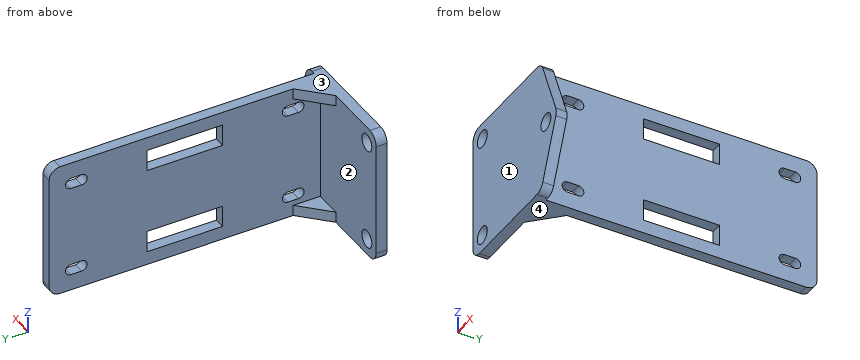
Autodesk Inventor part; units mm, degrees
ref_plane "YZ Plane" through (0, 0, 0) normal (1, 0, 0) x (0, 1, 0)
ref_plane "XZ Plane" through (0, 0, 0) normal (0, 1, 0) x (-1, 0, 0)
ref_plane "XY Plane" through (0, 0, 0) normal (0, 0, 1) x (1, 0, 0)
sketch "Sketch1" plane through (0, 0, 0) normal (0, 1, 0) x (-1, 0, 0)
  line L0 (-10, -12.5) -> (-10, 12.5)
  line L1 (-10, 12.5) -> (10, 12.5)
  line L2 (10, 12.5) -> (10, -12.5)
  line L3 (10, -12.5) -> (-10, -12.5)
  line L4 (-10, -12.5) -> (10, 12.5) construction
  line L5 (-10, 12.5) -> (10, -12.5) construction
  line L6 (-10, -12.5) -> (-10.6459, -12.5)
  line L7 (-10, 12.5) -> (-10.6459, 12.5)
  line L8 (-16.7029, -0.7428) -> (-12.5029, -11.2428)
  line L9 (-12.5029, 11.2428) -> (-16.7029, 0.7428)
  circle A0 centre (-13.5, 0) radius 1.6
  arc A1 (-16.7029, 0.7428) -> (-16.7029, -0.7428) centre (-14.8459, 0) ccw
  arc A2 (-10.6459, 12.5) -> (-12.5029, 11.2428) centre (-10.6459, 10.5) ccw
  arc A3 (-12.5029, -11.2428) -> (-10.6459, -12.5) centre (-10.6459, -10.5) ccw
  point P0 (0, 0)
  point P1 (-12, -12.5)
  point P2 (-12, 12.5)
  dimension "d1" = 20
  dimension "d63" = 2
  dimension "d64" = 2
  dimension "d66" = 3.2
  dimension "d67" = 2
extrude "Extrusion1" add sketch "Sketch1" along normal blind 2
sketch "Sketch2" plane through (0, 2, 0) normal (0, 1, 0) x (1, 0, 0)
  line L0 (10, 12.5) -> (10, -12.5)
  line L1 (10, -12.5) -> (8, -12.5)
  line L2 (8, -12.5) -> (8, 12.5)
  line L3 (8, 12.5) -> (10, 12.5)
  line L4 (10, -12.5) -> (10, 12.5)
  point P0 (0, 0)
  dimension "d4" = 2
extrude "Extrusion2" add sketch "Sketch2" along normal blind 50
sketch "Sketch3" plane through (8, 2, -12.5) normal (-1, 0, 0) x (0, 0, 1)
  line L0 (0, 0) -> (25, 0)
  line L1 (2.5, 2.5) -> (2.5, 47.5)
  line L2 (2.5, 47.5) -> (22.5, 47.5)
  line L3 (22.5, 47.5) -> (22.5, 2.5)
  line L4 (22.5, 2.5) -> (2.5, 2.5)
  line L5 (2.5, 2.5) -> (4, 2.5)
  line L6 (22.5, 2.5) -> (21, 2.5)
  line L7 (22.5, 25) -> (22.5, 32)
  line L8 (22.5, 32) -> (18.5, 32)
  line L9 (18.5, 32) -> (18.5, 18)
  line L10 (18.5, 18) -> (22.5, 18)
  line L11 (2.5, 25) -> (2.5, 32)
  line L12 (2.5, 32) -> (6.5, 32)
  line L13 (6.5, 32) -> (6.5, 18)
  line L14 (6.5, 18) -> (2.5, 18)
  line L15 (3, 46) -> (3, 44)
  line L16 (5, 46) -> (5, 44)
  arc A0 (5, 46) -> (3, 46) centre (4, 46) ccw
  arc A1 (3, 44) -> (5, 44) centre (4, 44) ccw
  line L17 (20, 46) -> (20, 44)
  line L18 (22, 46) -> (22, 44)
  arc A2 (22, 46) -> (20, 46) centre (21, 46) ccw
  arc A3 (20, 44) -> (22, 44) centre (21, 44) ccw
  line L19 (3, 6) -> (3, 4)
  line L20 (5, 6) -> (5, 4)
  arc A4 (5, 6) -> (3, 6) centre (4, 6) ccw
  arc A5 (3, 4) -> (5, 4) centre (4, 4) ccw
  line L21 (20, 6) -> (20, 4)
  line L22 (22, 6) -> (22, 4)
  arc A6 (22, 6) -> (20, 6) centre (21, 6) ccw
  arc A7 (20, 4) -> (22, 4) centre (21, 4) ccw
  point P0 (12.5, -2)
  point P1 (2.5, 43)
  point P2 (22.5, 43)
  point P3 (2.5, 7)
  point P4 (22.5, 7)
  dimension "d10" = 45
  dimension "d11" = 20
  dimension "d42" = 4
  dimension "d43" = 14
  dimension "d44" = 2
  dimension "d45" = 2
  dimension "d46" = 2
  dimension "d47" = 2
  dimension "d48" = 2
  dimension "d49" = 2
  dimension "d50" = 2
  dimension "d51" = 2
extrude "Extrusion3" cut sketch "Sketch3" against normal blind 2 contours L1 L12 L13 L14 | L10 L9 L8 L3 | A0 L16 A1 L15 | A2 L18 A3 L17 | A4 L20 A5 L19 | A6 L22 A7 L21
sketch "Sketch5" plane through (0, 2, 0) normal (0, 1, 0) x (1, 0, 0)
  line L0 (10.6459, 12.5) -> (-10, 12.5)
  line L1 (8, 12.5) -> (3, 12.5)
  line L2 (3, 12.5) -> (3, 10.5)
  line L3 (3, 10.5) -> (8, 10.5)
  line L4 (8, 10.5) -> (8, 12.5)
  line L5 (-10, -12.5) -> (8, -12.5)
  line L6 (8, -12.5) -> (3, -12.5)
  line L7 (3, -12.5) -> (3, -10.5)
  line L8 (3, -10.5) -> (8, -10.5)
  line L9 (8, -10.5) -> (8, -12.5)
  point P0 (0, 0)
  point P1 (10, 12.5)
  point P2 (10.9055, 12.5)
  dimension "d22" = 5
  dimension "d23" = 2
  dimension "d24" = 5
  dimension "d25" = 2
extrude "Extrusion4" add sketch "Sketch5" along normal blind 5
chamfer "Chamfer1" distance 5 angle 45 2 edges at (3, 7, -11.5) (3, 7, 11.5)
sketch "Sketch6" plane through (0, 2, 0) normal (0, 1, 0) x (1, 0, 0)
  line L0 (-10, -12.5) -> (-7, -12.5)
  line L1 (-10, -12.5) -> (3, -12.5)
  line L2 (-7, -12.5) -> (-7, -9.5)
  circle A0 centre (-7, -9.5) radius 1.6
  line L3 (-10, 12.5) -> (-7, 12.5)
  line L4 (3, 12.5) -> (-10, 12.5)
  line L5 (-7, 12.5) -> (-7, 9.5)
  circle A1 centre (-7, 9.5) radius 1.6
  point P0 (0, 0)
  dimension "d31" = 3
  dimension "d32" = 3
  dimension "d33" = 3.2
  dimension "d34" = 3
  dimension "d35" = 3
  dimension "d36" = 3.2
extrude "Extrusion5" cut sketch "Sketch6" against normal blind 5
fillet "Fillet1" radius 2 4 edges at (-10, 1, 12.5) (-10, 1, -12.5) (9, 52, 12.5) (9, 52, -12.5)
equation "\"d20\" = d49"
properties part number "Sonar Mount" material "ABS Plastic"
Input: part model. Units: mm. Frame: model coordinates. Face numbers are marked on the shaded views. Coordinates: 2 decimals unless noted, no trailing zeros. Loops run counter-clockwise (first coordinate to the right, second up) from the corner with the lowest first, then second, coordinate; pieces in that order, holes last.
Q1. Material intervals for line 1 (Z direction, x = -7, y = 1.4); line 2 (Z direction, x = 8.25, y = 31); line 3 (X direction, y = 11.5, z = -3), sorted ascending.
Q2. Contact query for flat-ended pins moving along their axis: pin 1 (1.5 mm diameter, centred on x = 6, y = 5.5, fed in from +Z); pin 2 (5 mm diameter, centred on x = -7, z = -9.5, fed in from +Y); pin 3 (6 mm diameter, centred on y = 17, z = -7.5, fed in from -X); pin 4 (6 mm diameter, centred on y = 7, z = 3, fed in from +X). Output: stop coordinate, or through.
Q3. Cut plane D-D (z = 8.5). Output: boundary loops of the cut face in (x, y), then the cut area to 3 significant figures.
Q4. Cut plane C-C (x = 9). Give the number of separate pieces and of enclosed holes in the cut face, then the cut area to 3 significant figures.
Q5. Cut plane A-A (y = 30.5). Output: boundary loops of the cut face in (x, z).
Q6. Cut plane B-B (x = -7). Output: boundary loops of the cut face in (y, z), then the cut area to 3 significant figures.
Q7. Draft query along Z for the marked faces 1, 2, 3 and 4. Return one class per face: +Z half, -Z half, draft (parallel to the pull), parting line (faces both ways), or undercut.
Working result:
1. line 1: z = -12.5 to -11.1, -7.9 to 7.9, 11.1 to 12.5
1. line 2: z = -12.5 to -10, -6 to 6, 10 to 12.5
1. line 3: x = 8 to 10
2. pin 1: stops at z = 12.5
2. pin 2: stops at y = 2
2. pin 3: stops at x = 8
2. pin 4: stops at x = 10
3. outline: (-10, 0) - (-8.25, 0) - (-8.25, 2) - (-10, 2) - close; (-5.75, 0) - (13.6, 0) - (13.6, 2) - (10, 2) - (10, 5) - (8, 5) - (8, 2) - (-5.75, 2) - close; (8, 9) - (10, 9) - (10, 20) - (8, 20) - close; (8, 34) - (10, 34) - (10, 45) - (8, 45) - close; (8, 49) - (10, 49) - (10, 52) - (8, 52) - close
3. area: 98.2 mm2
4. separate pieces: 1
4. enclosed holes: 6
4. area: 1,160 mm2
5. outline: (8, -12.5) - (10, -12.5) - (10, -10) - (8, -10) - close; (8, -6) - (10, -6) - (10, 6) - (8, 6) - close; (8, 10) - (10, 10) - (10, 12.5) - (8, 12.5) - close
6. outline: (0, -12.5) - (2, -12.5) - (2, -11.1) - (0, -11.1) - close; (0, -7.9) - (2, -7.9) - (2, 7.9) - (0, 7.9) - close; (0, 11.1) - (2, 11.1) - (2, 12.5) - (0, 12.5) - close
6. area: 37.2 mm2
7. face 1: draft
7. face 2: undercut
7. face 3: +Z half
7. face 4: -Z half
